```python
from build123d import *

# Parameters (mm, degrees)
F0_W     = 25.4
F0_H     = 25.4
F0_W_2   = 21.844
F0_H_2   = 21.844
F1_DEPTH = 88.9
F2_R     = 2.4892
F3_DEPTH = 25.4
F4_R     = 2.4892
F5_DEPTH = 1.778


with BuildPart() as f1:
    # F0 (on Front) → F1 (new body)
    with BuildSketch(Plane.XZ):
        with Locations((-12.7, 12.7)):
            Rectangle(F0_W, F0_H)
        with Locations((-12.7, 12.7)):
            Rectangle(F0_W_2, F0_H_2, mode=Mode.SUBTRACT)
    extrude(amount=F1_DEPTH)

    # F2 (on face) → F3 (cut)
    with BuildSketch(Plane(origin=(-25.4, 0, 0), x_dir=(0, -1, 0), z_dir=(-1, 0, 0))):
        with Locations((12.7, 19.05)):
            Circle(F2_R)
        with Locations((25.4, 19.05)):
            Circle(F2_R)
        with Locations((38.1, 19.05)):
            Circle(F2_R)
        with Locations((50.8, 19.05)):
            Circle(F2_R)
        with Locations((63.5, 19.05)):
            Circle(F2_R)
        with Locations((76.2, 19.05)):
            Circle(F2_R)
    extrude(amount=-F3_DEPTH, mode=Mode.SUBTRACT)

    # F4 (on face) → F5 (cut, through all)
    with BuildSketch(Plane(origin=(0, 0, 0), x_dir=(1, 0, 0), z_dir=(0, 0, -1))):
        with Locations((-12.7, 76.2)):
            Circle(F4_R)
        with Locations((-12.7, 63.5)):
            Circle(F4_R)
        with Locations((-12.7, 50.8)):
            Circle(F4_R)
        with Locations((-12.7, 38.1)):
            Circle(F4_R)
        with Locations((-12.7, 25.4)):
            Circle(F4_R)
        with Locations((-12.7, 12.7)):
            Circle(F4_R)
    extrude(amount=-F5_DEPTH, mode=Mode.SUBTRACT)


solid = f1.part
```
Could you check a few things on this model? Use its own coordinates, in mm. A direction names the side the tool comes from. Round coordinates to 2 decimals unless told otherwise and drop trailing zeros. Loops run counter-clockwise (first coordinate to the right, second up) from the corner with the lowest first, then second, coordinate; pieces in that order, holes last. Notation, with made-up numbers: M 37,85.25 L 81,85.25 A15 cw 81,93.25 Z; hole C -34.75,-22 d11. An arc over 180 degrees is marked long. Write item = value, one per line.
1. I want a section at D-D, the plane x = -17.5. Write out the boundary of the cut face in (y, z).
Results below:
outline = M -88.9,0 L 0,0 L 0,1.78 L -88.9,1.78 Z; M -88.9,23.62 L 0,23.62 L 0,25.4 L -88.9,25.4 Z
2. I want a section at C-C, the plane z = 13. Write out the boundary of the cut face in (x, y).
Results below:
outline = M -25.4,-88.9 L -23.62,-88.9 L -23.62,0 L -25.4,0 Z; M -1.78,-88.9 L 0,-88.9 L 0,0 L -1.78,0 Z
3. I need wall thicknesses on probe 1 along X at (y, z) = (-79, 3.25); probe 2 along Z at (x, y) = (-18.25, -46); probe 3 along X at (y, z) = (-50.8, 1.1). Which ranges of each line are inside material? Lowest first, please.
Results below:
probe_1 = -25.4 to -23.62, -1.78 to 0
probe_2 = 0 to 1.78, 23.62 to 25.4
probe_3 = -25.4 to -15.19, -10.21 to 0
4. I want a section at B-B, the plane y = -30.5. Write out the boundary of the cut face in (x, z), and give its area (3 significant figures).
Results below:
outline = M -25.4,0 L 0,0 L 0,25.4 L -25.4,25.4 Z; hole M -23.62,1.78 L -1.78,1.78 L -1.78,23.62 L -23.62,23.62 Z
area = 168 mm²
5. Which directions (+Z, -Z, +X, -X, +Y, -Y) give clear straight access to the entire face, cutting with the end or side of a thin tool? Please do faces 1 (the face through (-24.523, -35.613, 19.159)), 2 (the face through (-13.02, -53.27, 0.88)), 3 (the face through (-13, -44, 23.622)).
Results below:
face_1 = +X, -X
face_2 = -Z
face_3 = +Y, -Y
6. Will these pins go through, and if not, where does the flat tip stop? P1, Ø4, axis at y = -76.2, z = 19.05, coming from the -X side; P2, Ø4, axis at x = -12.7, y = -76.2, coming from the -Z side.
Results below:
P1 = through
P2 = 23.62
7. I want a section at A-A, the plane x = -12.7. Count the separate pieces of the cut face and the enclosed holes in it, and give its area (3 significant figures).
Results below:
separate_pieces = 8
enclosed_holes = 0
area = 263 mm²
8. Thinking about a two-plate mould opening in X: for faces 4 (the face through (-0.9, -53.1, 18.1)), 5 (the face through (-11.36, -65.6, 0.88)), 6 (the face through (-13, -44, 1.778)), 7 (the face through (-25.4, -44, 13)), which applies, +X half, -X half, draft (parallel to the pull), parting line (faces both ways), or undercut?
Results below:
face_4 = draft
face_5 = undercut
face_6 = undercut
face_7 = -X half
